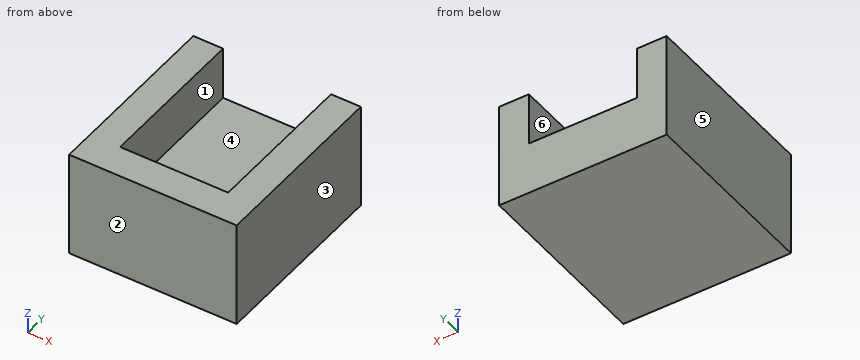
```python
from build123d import *

# Parameters (mm, degrees)
F0_W     = 12.4
F0_H     = 18.5
F1_DEPTH = 6.35
F2_W     = 12.4
F2_H     = 12.7
F3_DEPTH = 3.81
F4_W     = 22.31
F4_H     = 12.7
F5_DEPTH = 3.81
F6_W     = 22.31
F6_H     = 12.7
F7_DEPTH = 3.81
F8_W     = 12.908
F8_H     = 18.5
F9_DEPTH = 6.35


with BuildPart() as f1:
    # F0 (on Top) → F1 (new body)
    with BuildSketch(Plane.XY):
        with Locations((-3.637616, -16.132845)):
            Rectangle(F0_W, F0_H)
    extrude(amount=F1_DEPTH)

    # F2 (on face) → F3 (join)
    with BuildSketch(Plane.XZ.offset(25.382845)):
        with Locations((-3.637616, 6.35)):
            Rectangle(F2_W, F2_H)
    extrude(amount=F3_DEPTH)

    # F4 (on face) → F5 (join)
    with BuildSketch(Plane.YZ.offset(2.562384)):
        with Locations((-18.037845, 6.35)):
            Rectangle(F4_W, F4_H)
    extrude(amount=F5_DEPTH)

    # F6 (on face) → F7 (join)
    with BuildSketch(Plane(origin=(-9.837616, 0, 0), x_dir=(0, -1, 0), z_dir=(-1, 0, 0))):
        with Locations((18.037845, 6.35)):
            Rectangle(F6_W, F6_H)
    extrude(amount=F7_DEPTH)

    # F8 (on face) → F9 (cut, through all)
    with BuildSketch(Plane.XY.offset(12.7)):
        with Locations((-3.637616, -16.132845)):
            Rectangle(F8_W, F8_H)
    extrude(amount=-F9_DEPTH, mode=Mode.SUBTRACT)


solid = f1.part
```
Here's how the part is built. I have some questions about the finished solid (model axes, mm). Face numbers are marked on the shaded views. A direction names the side the tool comes from. Coordinates: 2 decimals unless noted, no trailing zeros. Loops run counter-clockwise (first coordinate to the right, second up) from the corner with the lowest first, then second, coordinate; pieces in that order, holes last. Notation, with made-up numbers: (0.5, -6) - (36.5, -6) arc R26 cw to (36.5, 31) - close; hole circle Ø2 at (64, 49). An arc over 180 degrees is marked (long way). Return JSON: item names as keys, results as strings. Group by question number.
Item 1: Will these pins go through, and if not, where does the flat tip stop? P1, Ø4, axis at x = 0, z = 8.5, coming from the +Y side; P2, Ø10.5, axis at x = -3, y = -11.5, coming from the +Z side.
Item 2: We'd pull the mould along X, two halves only. Please class the marked faces 3, 4, 5 and 6: +X half, -X half, draft (parallel to the pull), parting line (faces both ways), or undercut.
Item 3: If we section it at C-C on x = 2.25: Write out the boundary of the cut face in (y, z).
Item 4: On a 3-axis mill with a long thin cutter (end or side, diameter ignored), from which of +Z, -Z, +X, -X, +Y, -Y can I reach the whole of each face in a straight line? I mean the marked faces 1 and 2. Say none if no direction works.
Item 5: I need wall thicknesses on line 1 (X direction, y = -18, z = 6.5); line 2 (Y direction, x = -7.25, z = 6.5); line 3 (Z direction, x = 1.5, y = -17.5). Which ranges of each line are inside material? Lowest first, please. Write a range as from..to.
Item 6: If we section it at B-B on y = -19: Write out the boundary of the cut face in (x, z), and give its area (3 significant figures).
Item 7: If we section it at A-A on z = 7.5: Write out the boundary of the cut face in (x, y).
Calculated:
{
 "1": {"P1": "stops at y = -25.38", "P2": "stops at z = 6.35"},
 "2": {"face 3": "+X half", "face 4": "undercut", "face 5": "-X half", "face 6": "undercut"},
 "3": {"outline": "(-29.19, 0) - (-6.88, 0) - (-6.88, 6.35) - (-25.38, 6.35) - (-25.38, 12.7) - (-29.19, 12.7) - close"},
 "4": {"face 1": "+Z, +Y", "face 2": "+Z, -Z, +X, -X, -Y"},
 "5": {"line 1": "x = -13.65..-10.09, 2.82..6.37", "line 2": "y = -29.19..-25.38", "line 3": "z = 0..6.35"},
 "6": {"outline": "(-13.65, 0) - (6.37, 0) - (6.37, 12.7) - (2.82, 12.7) - (2.82, 6.35) - (-10.09, 6.35) - (-10.09, 12.7) - (-13.65, 12.7) - close", "area": "172 mm^2"},
 "7": {"outline": "(-13.65, -29.19) - (6.37, -29.19) - (6.37, -6.88) - (2.82, -6.88) - (2.82, -25.38) - (-10.09, -25.38) - (-10.09, -6.88) - (-13.65, -6.88) - close"}
}
